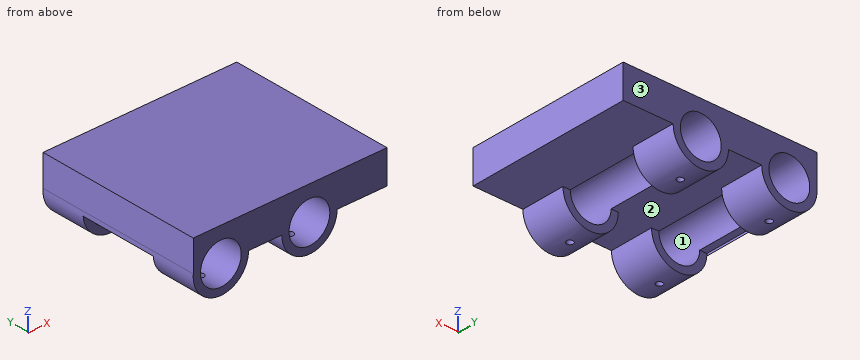
```python
from build123d import *

# Parameters (mm, degrees)
F0_W        = 70
F0_H        = 60
F1_DEPTH    = 12
F3_DEPTH    = 60.001
F2_R        = 10
F2_R_2      = 7.375
F4_DEPTH    = 60
F6_W        = 14
F6_H        = 16.388628301
F7_DEPTH    = 70.001
F10_D       = 2.4
F10_DEPTH   = 10
F10_START   = 0.0740526
F10_START_2 = 0.1005893
F10_TIP     = 0.7210327428


with BuildPart() as f1:
    # F0 (on Top) → F1 (new body)
    with BuildSketch(Plane.XY):
        Rectangle(F0_W, F0_H)
    extrude(amount=F1_DEPTH)

    # F2 (on face) → F3 (cut, through all)
    with BuildSketch(Plane.XZ.offset(30)):
        with BuildLine():
            Line((-32.4059612602, 0), (-17.6559612602, 0))
            ThreePointArc((-17.6559612602, 0), (-25.0309612602, 7.375), (-32.4059612602, 0))
        make_face()
        with BuildLine():
            ThreePointArc((14.3440387398, 0), (6.9690387398, 7.375), (-0.4059612602, 0))
            Line((-0.4059612602, 0), (14.3440387398, 0))
        make_face()
    extrude(amount=-F3_DEPTH, mode=Mode.SUBTRACT)

    # F2 (on face) → F4 (join, through all)
    with BuildSketch(Plane.XZ.offset(30)):
        with Locations((-25.0309612602, 0)):
            Circle(F2_R)
        with Locations((-25.0309612602, 0)):
            Circle(F2_R_2, mode=Mode.SUBTRACT)
        with Locations((6.9690387398, 0)):
            Circle(F2_R)
        with Locations((6.9690387398, 0)):
            Circle(F2_R_2, mode=Mode.SUBTRACT)
    extrude(amount=-F4_DEPTH)

    # F6 (on offset) → F7 (cut, through all)
    with BuildSketch(Plane(origin=(-35, 0, 0), x_dir=(0, -1, 0), z_dir=(-1, 0, 0))):
        with Locations((-7, -8.1943141505)):
            Rectangle(F6_W, F6_H)
        with Locations((7, -8.1943141505)):
            Rectangle(F6_W, F6_H)
    extrude(amount=-F7_DEPTH, mode=Mode.SUBTRACT)

    # F10
    # its depths count from where the whole tool has entered the part; down to there all is cleared
    with Locations(Plane(origin=(0, 0, -10), x_dir=(1, 0, 0), z_dir=(0, 0, -1))):
        with Locations((-25.0456897311, -21.936209172, -F10_START), (7.1838408707, -22.0174100382, -F10_START_2), (7.1838408707, 22.0174100382, -F10_START_2), (-25.0456897311, 21.936209172, -F10_START)):
            Hole(F10_D / 2, depth=F10_DEPTH)
            with Locations((0, 0, -(F10_DEPTH + F10_TIP / 2))):  # 118° drill point
                Cone(0, F10_D / 2, F10_TIP, mode=Mode.SUBTRACT)


solid = f1.part
```
Work out the finished part from the listing and answer in its coordinate system (mm). Face numbers are marked on the shaded views. Round coordinates to 2 decimals unless told otherwise and drop trailing zeros. Loops run counter-clockwise (first coordinate to the right, second up) from the corner with the lowest first, then second, coordinate; pieces in that order, holes last.
(1) The part is cut by section A-A, the plane y = -6.5. Give the vertices of the cut face in (x, z) (3 decimals), and give its area (3 significant figures).
Computed values:
outline: (-35, -0.786) - (-35, 0) - (-32.406, 0) arc R7.375 cw to (-17.656, 0) - (-0.406, 0) arc R7.375 cw to (14.344, 0) - (35, 0) - (35, 12) - (-35, 12) - (-35, 0.786) arc R10 ccw to start
area: 669 mm2
(2) The part is cut by section D-D, the plane y = 16. Give the vertices of the cut face in (x, z) (3 decimals).
Computed values:
outline: (-35, 0.786) arc R10 ccw (long way) to (-15.031, 0) - (-3.031, 0) arc R10 ccw to (16.969, 0) - (35, 0) - (35, 12) - (-35, 12) - close; hole circle Ø14.75 at (-25.031, 0); hole circle Ø14.75 at (6.969, 0)
(3) The mould has two halves that part along Z. Classify the marked faces 1, 2 and 3: pulls with the +Z half, pulls with the -Z half, needs draft (parallel to the pull), parting line crosses it, or undercut.
Computed values:
face 1: undercut
face 2: pulls with the -Z half
face 3: needs draft
(4) Find the intervals of material crossed by L1, parallel to X at y = 21.5, z = 0.5; L2, parallel to X at y = -23, z = -7.75; L3, parallel to X at y = -23.5, z = 6, in increasing order.
Computed values:
L1: x = -35.02 to -32.39, -17.67 to -0.39, 14.33 to 35
L2: x = -31.35 to -25.6, -24.49 to -18.71, 0.65 to 6.49, 7.87 to 13.29
L3: x = -35 to -29.32, -20.74 to 2.68, 11.26 to 35
(5) The part is cut by section B-B, the plane z = -2. Give the number of separate pieces and of enclosed holes in the cut face, and give its area (3 significant figures).
Computed values:
separate pieces: 8
enclosed holes: 0
area: 346 mm2
(6) Each of these flat-tipped pins is pushed along its axis until it touches: P1, Ø9, axis at x = -25.03, z = 0, coming from the +Y side; P2, Ø16.5, axis at x = 26.5, y = 1, coming from the -Z side; P3, Ø6, axis at y = -22.5, z = -5, coming from the -X side; P4, Ø3, axis at x = -24.5, y = 8, coming from the -Z side. Where does it stop, or does it pass through?
Computed values:
P1: passes through
P2: stops at z = 0
P3: stops at x = -34.83
P4: stops at z = 7.09
(7) The part is cut by section C-C, the plane x = 10.5. Give the vertices of the cut face in (y, z).
Computed values:
outline: (-30, -9.36) - (-14, -9.36) - (-14, -6.47) - (-30, -6.47) - close; (-30, 6.47) - (30, 6.47) - (30, 12) - (-30, 12) - close; (14, -9.36) - (30, -9.36) - (30, -6.47) - (14, -6.47) - close
